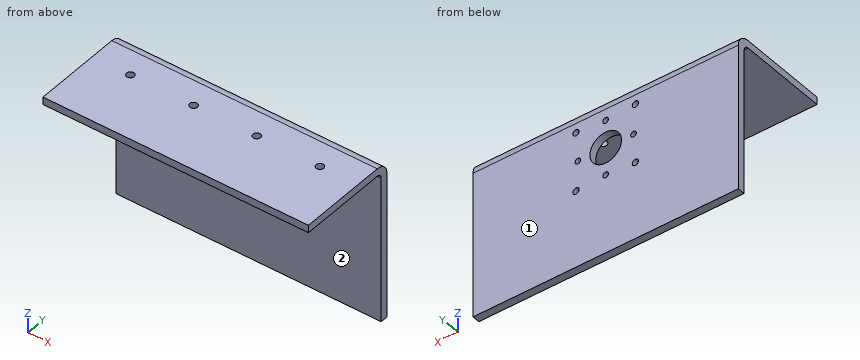
```python
from build123d import *

# Parameters (mm, degrees)
BASE_FLANGE1_DEPTH = 105
SKETCH6_R          = 12.5
SKETCH6_R_2        = 2.5
CUT_EXTRUDE1_DEPTH = 10
SKETCH7_R          = 3
CUT_EXTRUDE2_DEPTH = 10
SKETCH8_R          = 2.25
CUT_EXTRUDE3_DEPTH = 10


# Sheet-metal steps are written as plain solids
with BuildPart() as part:
    # Sketch1 → Base-Flange1 (new, symmetric)
    with BuildSketch(Plane(origin=(0, 0, 0), x_dir=(0, 0, -1), z_dir=(1, 0, 0))):
        with BuildLine():
            Line((0, -75), (0, -4))
            ThreePointArc((0, -4), (1.171572875, -1.171572875), (4, 0))
            Line((4, 0), (120, 0))
            Line((120, 0), (120, 6))
            Line((120, 6), (4, 6))
            ThreePointArc((4, 6), (-3.071067812, 3.071067812), (-6, -4))
            Line((-6, -4), (-6, -75))
            Line((-6, -75), (0, -75))
        make_face()
    extrude(amount=BASE_FLANGE1_DEPTH, both=True)

    # Sketch6 → Cut-Extrude1 (cut)
    with BuildSketch(Plane(origin=(0, 6, 0), x_dir=(1, 0, 0), z_dir=(0, 1, 0))):
        with Locations(Location((0, 35, 0), (0, 0, 270))):
            Circle(SKETCH6_R)
        with Locations(Location((23.5, 58.5, 0), (0, 0, 270))):
            Circle(SKETCH6_R_2)
        with Locations(Location((-23.5, 58.5, 0), (0, 0, 270))):
            Circle(SKETCH6_R_2)
        with Locations(Location((-23.5, 11.5, 0), (0, 0, 270))):
            Circle(SKETCH6_R_2)
        with Locations(Location((23.5, 11.5, 0), (0, 0, 270))):
            Circle(SKETCH6_R_2)
    extrude(amount=-CUT_EXTRUDE1_DEPTH, mode=Mode.SUBTRACT)

    # Sketch7 → Cut-Extrude2 (cut)
    with BuildSketch(Plane.XY.offset(6)):
        with Locations((-75, -24)):
            Circle(SKETCH7_R)
        with Locations((-25, -24)):
            Circle(SKETCH7_R)
        with Locations((25, -24)):
            Circle(SKETCH7_R)
        with Locations((75, -24)):
            Circle(SKETCH7_R)
    extrude(amount=-CUT_EXTRUDE2_DEPTH, mode=Mode.SUBTRACT)

    # Sketch8 → Cut-Extrude3 (cut)
    with BuildSketch(Plane(origin=(0, 6, 0), x_dir=(1, 0, 0), z_dir=(0, 1, 0))):
        with Locations(Location((0, 13, 0), (0, 0, 270))):
            Circle(SKETCH8_R)
        with Locations(Location((-22, 35, 0), (0, 0, 270))):
            Circle(SKETCH8_R)
        with Locations(Location((0, 57, 0), (0, 0, 270))):
            Circle(SKETCH8_R)
        with Locations(Location((22, 35, 0), (0, 0, 270))):
            Circle(SKETCH8_R)
    extrude(amount=-CUT_EXTRUDE3_DEPTH, mode=Mode.SUBTRACT)


solid = part.part
```
The listing builds one solid part. Answer for the finished solid, in the listing's coordinates (mm). Face numbers are marked on the shaded views. A direction names the side the tool comes from. Coordinates: 2 decimals unless noted, no trailing zeros. Loops run counter-clockwise (first coordinate to the right, second up) from the corner with the lowest first, then second, coordinate; pieces in that order, holes last. Notation, with made-up numbers: M 36,54.5 L 41,54.5 A29 cw 41,87.5 Z; hole C 51.5,65.5 d5. An arc over 180 degrees is marked long. Answer as a JSON object with one key per item and string values. Group by question number.
Item 1: Section A-A (z = -35) is taken. Write down the section's boundary in (x, y).
Item 2: Which of the six approach directions +Z, -Z, +X, -X, +Y, -Y give full straight-line access (tool end or side, diameter ignored) to the marked faces 1 and 2?
Item 3: Each of these flat-tipped pins is pushed along its axis until it touches: P1, Ø9.5, axis at x = 75, y = -24, coming from the +Z side; P2, Ø7, axis at x = -75, y = -24, coming from the -Z side; P3, Ø7, axis at x = -22, z = -35, coming from the -Y side. Where does it stop, or does it pass through?
Item 4: Section C-C (x = 75) is taken. Write down the section's boundary in (y, z).
Item 5: Consider L1, parallel to Z at x = -23, y = 3; L2, parallel to Y at x = 83.5, z = -23.5; L3, parallel to Y at x = -25, z = 2. Determine where each line is inside the solid, lowest interval first.
Item 6: Section B-B (x = 0) is taken. Write down the section's boundary in (y, z), and give its area (3 significant figures).
Item 7: Section D-D (x = 42.5) is taken. Write down the section's boundary in (y, z), and give its area (3 significant figures).
Solved:
{
 "1": {"outline": "M -105,0 L -24.25,0 L -24.25,6 L -105,6 Z; M -19.75,0 L -12.5,0 L -12.5,6 L -19.75,6 Z; M 12.5,0 L 19.75,0 L 19.75,6 L 12.5,6 Z; M 24.25,0 L 105,0 L 105,6 L 24.25,6 Z"},
 "2": {"face 1": "+Z, -Z, +X, -X, +Y", "face 2": "-Z, +X, -X, -Y"},
 "3": {"P1": "stops at z = 6", "P2": "stops at z = 0", "P3": "stops at y = 0"},
 "4": {"outline": "M -75,0 L -27,0 L -27,6 L -75,6 Z; M -21,0 L -4,0 A4 cw 0,-4 L 0,-120 L 6,-120 L 6,-4 A10 ccw -4,6 L -21,6 Z"},
 "5": {"L1": "z = -120 to -60.95, -56.05 to -37.02, -32.98 to -13.95, -9.05 to 3.14", "L2": "y = 0 to 6", "L3": "y = -75 to -27, -21 to 4"},
 "6": {"outline": "M -75,0 L -4,0 A4 cw 0,-4 L 0,-10.75 L 6,-10.75 L 6,-4 A10 ccw -4,6 L -75,6 Z; M 0,-120 L 6,-120 L 6,-59.25 L 0,-59.25 Z; M 0,-54.75 L 6,-54.75 L 6,-47.5 L 0,-47.5 Z; M 0,-22.5 L 6,-22.5 L 6,-15.25 L 0,-15.25 Z", "area": "984 mm2"},
 "7": {"outline": "M -75,0 L -4,0 A4 cw 0,-4 L 0,-120 L 6,-120 L 6,-4 A10 ccw -4,6 L -75,6 Z", "area": "1,190 mm2"}
}
